Drawing for the job (mm, zero at the part's lowest x, y, z). A direction names the side the tool comes from. Round coordinates to 2 decimals unless told otherwise and drop trailing zeros. Loops run counter-clockwise (first coordinate to the right, second up) from the corner with the lowest first, then second, coordinate; pieces in that order, holes last. Notation, with made-up numbers: (8, -14) -> (63, -14) arc R7 cw to (63, -4) -> close; hole circle Ø2 at (88.5, 84). An arc over 180 degrees is marked (long way). Put each result on its own line as item: value. Start each with the question number.
Item 1: Cut at A-A, the plane x = 2.55. List the corners of the cut face in (y, z), plus the area to 3 significant figures.
Item 2: Tool access for the marked faces 1 and 2: list every direction of +Z, -Z, +X, -X, +Y, -Y with a clear straight run to the whole face (end or side of a thin tool).
Item 3: Cut at B-B, the plane z = 3.85. List the corners of the cut face in (x, y).
Item 4: Flat gauge pins, fed straight in: pin 1 Ø1 at (x, y) = (1, 39) entering from -Z; pin 2 Ø1.5 at (x, y) = (4, 39) entering from +Z; pin 3 Ø2.5 at (x, z) = (3, 2.5) entering from -Y. Where does each tip first touch, or does it go through?
Item 5: Cut at C-C, the plane y = 10.5. List the corners of the cut face in (x, z).
Item 6: Drill centre lines: probe 1 along Y at (x, z) = (1.1, 5.75); probe 2 along Z at (x, y) = (3.5, 43.5). Where is each one in solid material? Low to high. Write a range as [from, to].
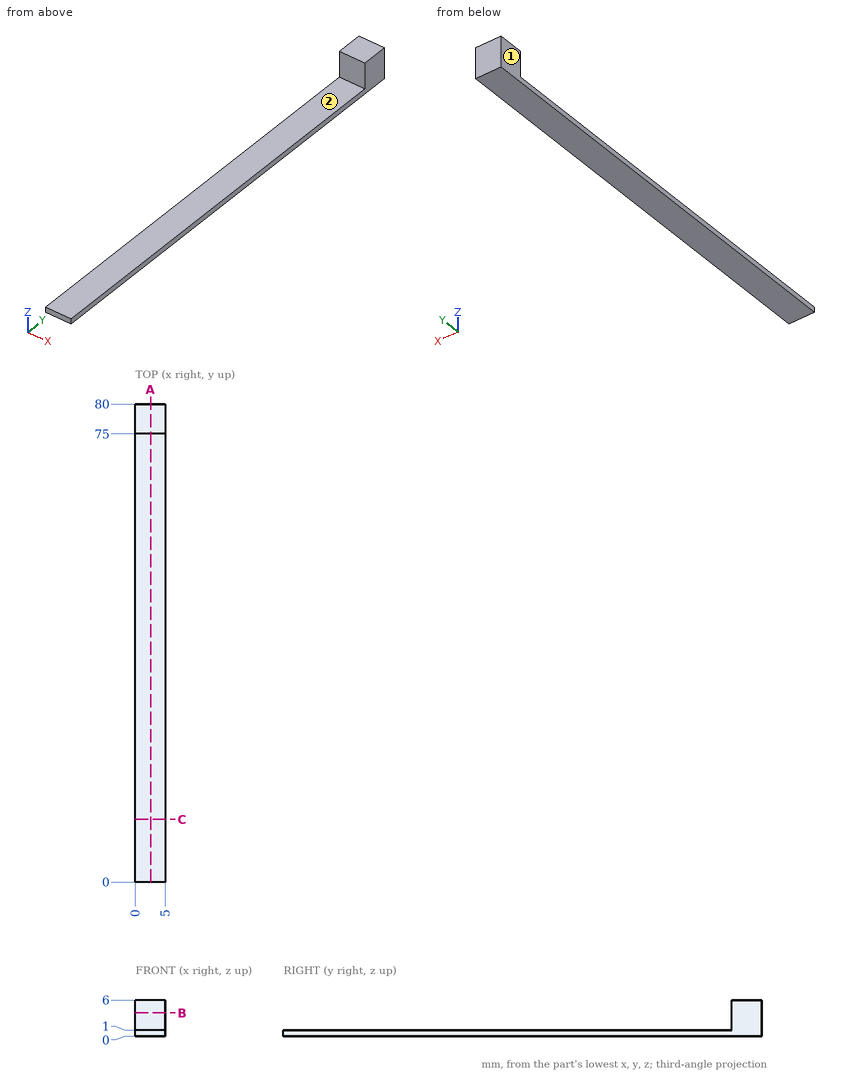
Reply:
1. outline: (0, 0) -> (80, 0) -> (80, 6) -> (75, 6) -> (75, 1) -> (0, 1) -> close
1. area: 105 mm^2
2. face 1: +Z, -Z, -X, +Y, -Y
2. face 2: +Z, +X, -X, -Y
3. outline: (0, 75) -> (5, 75) -> (5, 80) -> (0, 80) -> close
4. pin 1: stops at z = 0
4. pin 2: stops at z = 1
4. pin 3: stops at y = 75
5. outline: (0, 0) -> (5, 0) -> (5, 1) -> (0, 1) -> close
6. probe 1: y = [75, 80]
6. probe 2: z = [0, 1]
